Drawing for the job (mm, zero at the part's lowest x, y, z). A direction names the side the tool comes from. Give positions to 0.01 mm unless a question says otherwise; leave off trailing zeros. Loops run counter-clockwise (first coordinate to the right, second up) from the corner with the lowest first, then second, coordinate; pieces in that order, holes last.
1) Band-saw the part on D-D on x = 14.5. List the corners of the cut face in (y, z).
2) Band-saw the part on A-A on y = 16.5. List the corners of the cut face in (x, z), then the cut area to 3 significant figures.
3) Band-saw the part on C-C on z = 13. List the corners of the cut face in (x, y), then the cut area to 3 significant figures.
4) Two-plate mould, pull along Z, no slides. Class the marked faces 1, 2 and 3: +Z half, -Z half, draft (parallel to the pull), parting line (faces both ways), or undercut.
5) Band-saw the part on B-B on x = 11. List the corners of the cut face in (y, z).
6) Wall check: line 1 (Y direction, x = 20, z = 9.25); line 2 (Z direction, x = 20, y = 29); line 3 (X direction, y = 17, z = 1). Give the ranges that are in metal, low to high.
7) 3-axis set-ups, long thin cutter, end or side, ignore diameter. For the marked faces 4 and 5: which of +Z, -Z, +X, -X, +Y, -Y reach the whole face in a straight line?
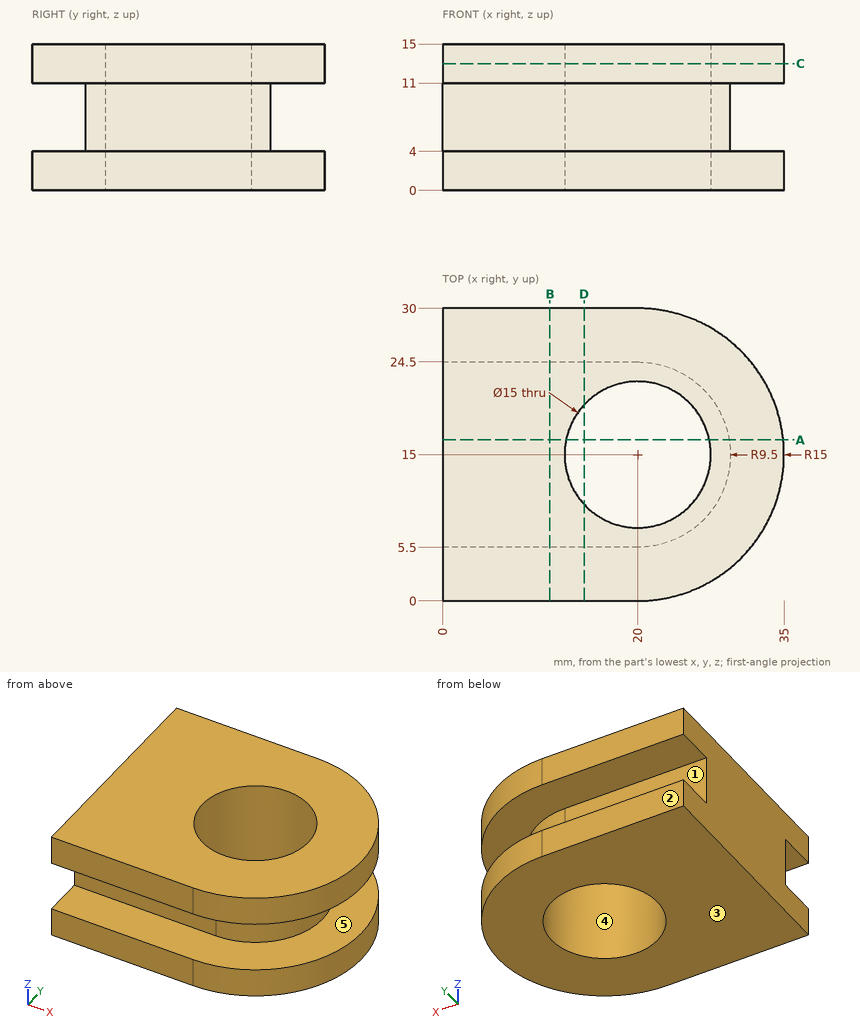
Findings below:
1. outline: (0, 0) - (9.9, 0) - (9.9, 15) - (0, 15) - (0, 11) - (5.5, 11) - (5.5, 4) - (0, 4) - close; (20.1, 0) - (30, 0) - (30, 4) - (24.5, 4) - (24.5, 11) - (30, 11) - (30, 15) - (20.1, 15) - close
2. outline: (0, 0) - (12.65, 0) - (12.65, 15) - (0, 15) - close; (27.35, 0) - (34.92, 0) - (34.92, 4) - (29.38, 4) - (29.38, 11) - (34.92, 11) - (34.92, 15) - (27.35, 15) - close
2. area: 265 mm2
3. outline: (0, 0) - (20, 0) arc R15 ccw to (20, 30) - (0, 30) - close; hole circle Ø15 at (20, 15)
3. area: 777 mm2
4. face 1: undercut
4. face 2: draft
4. face 3: -Z half
5. outline: (0, 0) - (30, 0) - (30, 4) - (24.5, 4) - (24.5, 11) - (30, 11) - (30, 15) - (0, 15) - (0, 11) - (5.5, 11) - (5.5, 4) - (0, 4) - close
6. line 1: y = 5.5 to 7.5, 22.5 to 24.5
6. line 2: z = 0 to 4, 11 to 15
6. line 3: x = 0 to 12.77, 27.23 to 34.87
7. face 4: +Z, -Z
7. face 5: +X
